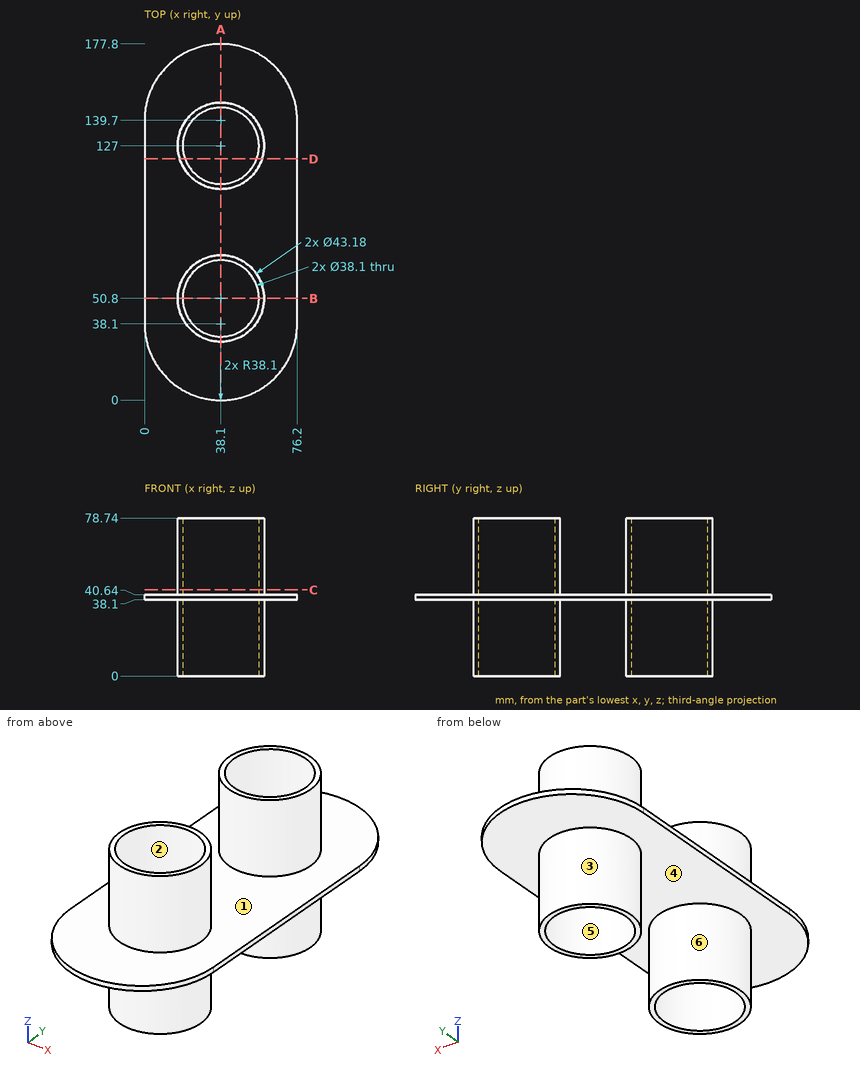
Study the drawing (mm; zero at the part's minimum x, y, z) and answer. A direction names the side the tool comes from. Coordinates: 2 decimals unless noted, no trailing zeros. Write each loop counter-clockwise with the first axis right and the second up, starting at its lowest first coordinate (ties: lowest second). Pieces come first, ordered by that corner, then holes.
Q1. Find the intervals of material crossed by line 1 (Y direction, x = 38.1, z = 58); line 2 (Y direction, x = 38, z = 40); line 3 (X direction, y = 50, z = 36), in increasing order.
Q2. Each of these flat-tipped pins is pushed along its axis until it touches: pin 1 Ø10 at (x, y) = (38, 28) entering from +Z; pin 2 Ø12 at (x, y) = (12.5, 82) entering from +Z; pin 3 Ø12 at (y, z) = (39, 52) entering from -X; pin 4 Ø10 at (x, z) = (41.5, 63.5) entering from -Y. Where does it stop, or does it pass through?
Q3. Which of the six approach directions +Z, -Z, +X, -X, +Y, -Y give full straight-line access (tool end or side, diameter ignored) to the marked faces 1, 2 and 3?
Q4. A cutting plane is placed at C-C, the plane z = 43. Give the vertices of the cut face in (x, y).
Q5. A cutting plane is placed at A-A, the plane x = 38.1. Give the vertices of the cut face in (y, z), then the cut area to 3 significant figures.
Q6. A cutting plane is placed at B-B, the plane y = 50.8. Give the vertices of the cut face in (x, z), then the cut area to 3 significant figures.
Q7. A cutting plane is placed at D-D, the plane y = 120.5. Give the vertices of the cut face in (x, z).
Q8. Determine the mould class of the marked faces 4, 5 and 6 for opening direction X: released by +X, released by -X, zero draft, split by the parting line, or undercut.
Findings below:
1. line 1: y = 29.21 to 31.75, 69.85 to 72.39, 105.41 to 107.95, 146.05 to 148.59
1. line 2: y = 0 to 31.75, 69.85 to 107.95, 146.05 to 177.8
1. line 3: x = 16.52 to 19.07, 57.13 to 59.68
2. pin 1: stops at z = 78.74
2. pin 2: stops at z = 40.64
2. pin 3: stops at x = 17.3
2. pin 4: stops at y = 29.21
3. face 1: +Z
3. face 2: +Z, -Z
3. face 3: -Z
4. outline: circle Ø43.18 at (38.1, 50.8); circle Ø43.18 at (38.1, 127); hole circle Ø38.1 at (38.1, 50.8); hole circle Ø38.1 at (38.1, 127)
5. outline: (0, 38.1) - (29.21, 38.1) - (29.21, 0) - (31.75, 0) - (31.75, 78.74) - (29.21, 78.74) - (29.21, 40.64) - (0, 40.64) - close; (69.85, 0) - (72.39, 0) - (72.39, 38.1) - (105.41, 38.1) - (105.41, 0) - (107.95, 0) - (107.95, 78.74) - (105.41, 78.74) - (105.41, 40.64) - (72.39, 40.64) - (72.39, 78.74) - (69.85, 78.74) - close; (146.05, 0) - (148.59, 0) - (148.59, 38.1) - (177.8, 38.1) - (177.8, 40.64) - (148.59, 40.64) - (148.59, 78.74) - (146.05, 78.74) - close
5. area: 1,030 mm2
6. outline: (0, 38.1) - (16.51, 38.1) - (16.51, 0) - (19.05, 0) - (19.05, 78.74) - (16.51, 78.74) - (16.51, 40.64) - (0, 40.64) - close; (57.15, 0) - (59.69, 0) - (59.69, 38.1) - (76.2, 38.1) - (76.2, 40.64) - (59.69, 40.64) - (59.69, 78.74) - (57.15, 78.74) - close
6. area: 484 mm2
7. outline: (0, 38.1) - (17.51, 38.1) - (17.51, 0) - (20.19, 0) - (20.19, 78.74) - (17.51, 78.74) - (17.51, 40.64) - (0, 40.64) - close; (56.01, 0) - (58.69, 0) - (58.69, 38.1) - (76.2, 38.1) - (76.2, 40.64) - (58.69, 40.64) - (58.69, 78.74) - (56.01, 78.74) - close
8. face 4: zero draft
8. face 5: undercut
8. face 6: split by the parting line
